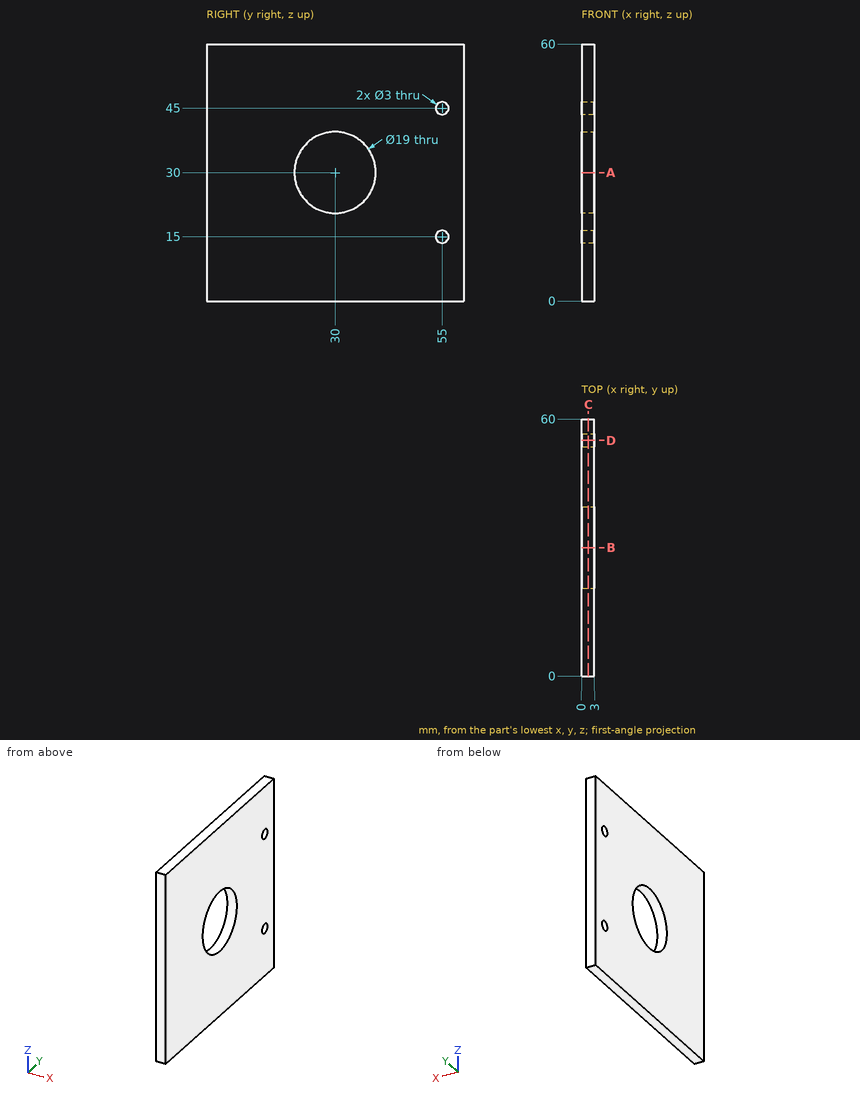
Geometry: see drawing. Coordinates: mm, zero at the bounding-box minimum. Coordinates: 2 decimals unless noted, no trailing zeros. Write each loop counter-clockwise with the first axis right and the second up, starting at its lowest first coordinate (ties: lowest second). Pieces come first, ordered by that corner, then holes.
1) Material intervals for line 1 along Y through (x, z) = (1.7, 15); line 2 along Z through (x, y) = (2.05, 38); line 3 along Z through (x, y) = (2.2, 29), sorted ascending.
2) Section C-C on x = 1.6. Output: boundary loops of the cut face in (y, z), and give its area (3 significant figures).
3) Pin query (flat end, axial travel): pin 1 Ø5 at (y, z) = (55, 45) entering from +X. Return the tip coordinate at first contact, or that it passes through.
4) Section A-A on z = 30. Output: boundary loops of the cut face in (x, y), and give its area (3 significant figures).
5) Section D-D on y = 55. Output: boundary loops of the cut face in (x, z), and give its area (3 significant figures).
Check result:
1. line 1: y = 0 to 53.5, 56.5 to 60
1. line 2: z = 0 to 24.88, 35.12 to 60
1. line 3: z = 0 to 20.55, 39.45 to 60
2. outline: (0, 0) - (60, 0) - (60, 60) - (0, 60) - close; hole circle Ø19 at (30, 30); hole circle Ø3 at (55, 15); hole circle Ø3 at (55, 45)
2. area: 3,300 mm2
3. pin 1: stops at x = 3
4. outline: (0, 0) - (3, 0) - (3, 20.5) - (0, 20.5) - close; (0, 39.5) - (3, 39.5) - (3, 60) - (0, 60) - close
4. area: 123 mm2
5. outline: (0, 0) - (3, 0) - (3, 13.5) - (0, 13.5) - close; (0, 16.5) - (3, 16.5) - (3, 43.5) - (0, 43.5) - close; (0, 46.5) - (3, 46.5) - (3, 60) - (0, 60) - close
5. area: 162 mm2
